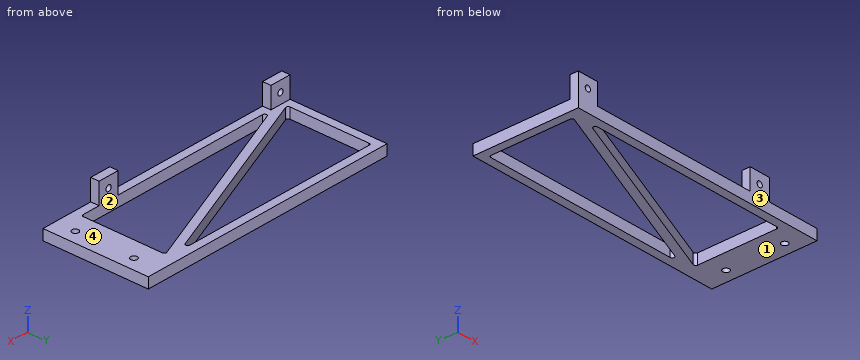
```python
from build123d import *

# Parameters (mm, degrees)
SKETCH_W     = 127
SKETCH_H     = 50.8
PAD_DEPTH    = 5.08
SKETCH001_R  = 1.5875
POCKET_DEPTH = 5.081
FILLET_R     = 0.999998
FILLET001_R  = 0.999998
FILLET002_R  = 0.999998
SKETCH002_W  = 10.16
SKETCH002_H  = 4.0132
PAD001_DEPTH = 10.16
SKETCH003_R  = 1.389063
HOLE_DEPTH   = 50.801


with BuildPart() as part:
    # Sketch → Pad (new body)
    with BuildSketch(Plane.XY):
        Rectangle(SKETCH_W, SKETCH_H)
    extrude(amount=PAD_DEPTH)

    # Sketch001 (on Face6 of Pad) → Pocket (cut, through all)
    with BuildSketch(Plane.XY.offset(5.08)):
        with Locations((57.15, 12.7)):
            Circle(SKETCH001_R)
        with Locations((57.15, -15.567334)):
            Circle(SKETCH001_R)
        Polygon((-54.077858, -21.3868), (47.585089, -21.3868), (47.585089, 19.226009), align=None)
        Polygon((42.176147, 21.3868), (-59.4868, 21.3868), (-59.4868, -19.226009), align=None)
    extrude(amount=-POCKET_DEPTH, mode=Mode.SUBTRACT)

    # Fillet
    fillet_edges = [part.edges().sort_by_distance(p)[0] for p in [
        (-59.4868, 21.3868, 2.54),
        (47.585089, -21.3868, 2.54),
    ]]
    fillet(fillet_edges, radius=FILLET_R)

    # Fillet001
    fillet001_edges = [part.edges().sort_by_distance(p)[0] for p in [
        (-54.077858, -21.3868, 2.54),
        (42.176147, 21.3868, 2.54),
    ]]
    fillet(fillet001_edges, radius=FILLET001_R)

    # Fillet002
    fillet002_edges = [part.edges().sort_by_distance(p)[0] for p in [
        (47.585089, 19.226009, 2.54),
        (-59.4868, -19.226009, 2.54),
    ]]
    fillet(fillet002_edges, radius=FILLET002_R)

    # Sketch002 (on Face20 of Fillet002) → Pad001 (join)
    with BuildSketch(Plane.XY.offset(5.08)):
        with Locations((-58.42, -23.3934)):
            Rectangle(SKETCH002_W, SKETCH002_H)
        with Locations((33.02, -23.3934)):
            Rectangle(SKETCH002_W, SKETCH002_H)
    extrude(amount=PAD001_DEPTH)

    # Sketch003 (on Face22 of Pad001) → Hole (cut, through all)
    with BuildSketch(Plane.XZ.offset(25.4)):
        with Locations((-58.42, 10.16)):
            Circle(SKETCH003_R)
        with Locations((33.02, 10.16)):
            Circle(SKETCH003_R)
    extrude(amount=-HOLE_DEPTH, mode=Mode.SUBTRACT)


solid = part.part
```
Input: part model. Units: mm. Frame: model coordinates. Face numbers are marked on the shaded views. A direction names the side the tool comes from. Coordinates: 2 decimals unless noted, no trailing zeros. Write each loop counter-clockwise with the first axis right and the second up, starting at its lowest first coordinate (ties: lowest second). Pieces come first, ordered by that corner, then holes. Notation, with made-up numbers: (62, 12) -> (91, 12) arc R17 cw to (91, 21) -> close; hole circle Ø5 at (61, -18.75). An arc over 180 degrees is marked (long way). Write each question's results on one line, items separated by ' | '.
Item 1: Section query A-A on x = 57.15. Return loops of the section in (y, z), plus the area to 3 significant figures.
Conclusion:
outline: (-25.4, 0) -> (-17.15, 0) -> (-17.15, 5.08) -> (-25.4, 5.08) -> close; (-13.98, 0) -> (11.11, 0) -> (11.11, 5.08) -> (-13.98, 5.08) -> close; (14.29, 0) -> (25.4, 0) -> (25.4, 5.08) -> (14.29, 5.08) -> close | area: 226 mm^2
Item 2: Section query D-D on z = 2.5. Count the separate pieces of the cut face and the enclosed holes in it, plus the area to 3 significant figures.
Conclusion:
separate pieces: 1 | enclosed holes: 4 | area: 2,320 mm^2
Item 3: Section query C-C on y = 12.7. Return loops of the section in (x, z), plus the area to 3 significant figures.
Conclusion:
outline: (-63.5, 0) -> (-59.49, 0) -> (-59.49, 5.08) -> (-63.5, 5.08) -> close; (20.43, 0) -> (31.25, 0) -> (31.25, 5.08) -> (20.43, 5.08) -> close; (47.59, 0) -> (55.56, 0) -> (55.56, 5.08) -> (47.59, 5.08) -> close; (58.74, 0) -> (63.5, 0) -> (63.5, 5.08) -> (58.74, 5.08) -> close | area: 140 mm^2
Item 4: Mould query, pull axis X, two halves, no side actions, for the marked faces 3 and 4. Classes: +X half, -X half, draft (parallel to the pull), parting line (faces both ways), or undercut.
Conclusion:
face 3: draft | face 4: undercut
Item 5: Pin query (flat end, axial travel): pin 1 Ø1 at (x, z) = (50, 7) entering from +Y; pin 2 Ø8 at (x, z) = (-60, 8.5) entering from +Y; pin 3 Ø3 at (x, z) = (-58.42, 10.16) entering from +Y; pin 4 Ø1.2 at (y, z) = (-22.5, 10.5) entering from +X. Return the tip coordinate at first contact, or that it passes through.
Conclusion:
pin 1: passes through | pin 2: stops at y = 25.4 | pin 3: stops at y = -21.39 | pin 4: stops at x = 38.1
Item 6: Material intervals for probe 1 along Y at (x, z) = (57.15, 3.75); probe 2 along X at (y, z) = (-22, 7.5); probe 3 along Z at (x, y) = (-58.42, -24.6), sorted ascending.
Conclusion:
probe 1: y = -25.4 to -17.15, -13.98 to 11.11, 14.29 to 25.4 | probe 2: x = -63.5 to -53.34, 27.94 to 38.1 | probe 3: z = 0 to 8.77, 11.55 to 15.24
Item 7: Set-up query: the marked faces 1 and 2. Return all of +Z, -Z, +X, -X, +Y, -Y with unobstructed straight access to the full face (end or side cutting, diameter ignored); none if empty.
Conclusion:
face 1: -Z, +X, -X, +Y, -Y | face 2: +Z, -Z
Item 8: Section query B-B on z = 7.5. Return loops of the section in (x, y).
Conclusion:
outline: (-63.5, -25.4) -> (-53.34, -25.4) -> (-53.34, -21.39) -> (-63.5, -21.39) -> close; (27.94, -25.4) -> (38.1, -25.4) -> (38.1, -21.39) -> (27.94, -21.39) -> close
